Autodesk Fusion 360 part; units mm, degrees
sketch "Sketch1" plane through (0, 0, 0) normal (0, 1, 0) x (1, 0, 0)
  line L0 (0, -1) -> (0, 0)
  line L1 (12, 0) -> (12, 1)
  line L2 (12, 1) -> (13, 1)
  line L3 (2, -1.5) -> (2, -2.5)
  line L4 (2, -2.5) -> (1, -2.5)
  line L5 (2, -1.5) -> (3, -1.5)
  line L6 (4.5, -1.5) -> (4.5, -8.5)
  line L7 (3, -8.5) -> (3, -1.5)
  line L8 (4.5, -1.5) -> (10.5, -1.5)
  line L9 (12, -1.5) -> (12, -8.5)
  line L10 (10.5, -8.5) -> (10.5, -1.5)
  line L11 (17.5, -10) -> (3, -10)
  line L12 (3, -10) -> (3, -8.5)
  line L13 (4.5, -8.5) -> (10.5, -8.5)
  line L14 (12, -8.5) -> (17.5, -8.5)
  line L15 (1, -2.5) -> (1, -1)
  line L16 (1, -1) -> (0, -1)
  line L17 (12, -1.5) -> (13, -1.5)
  line L18 (13, -1.5) -> (13, 1)
  line L19 (12, 0) -> (0, 0)
  line L20 (23, -1.5) -> (23, -8.5)
  line L21 (22, -1.5) -> (22, 1)
  line L22 (32, -8.5) -> (32, -1.5)
  line L23 (30.5, -8.5) -> (24.5, -8.5)
  line L24 (30.5, -1.5) -> (24.5, -1.5)
  line L25 (32, -10) -> (32, -8.5)
  line L26 (23, 0) -> (23, 1)
  line L27 (33, -1.5) -> (32, -1.5)
  line L28 (23, 1) -> (22, 1)
  line L29 (34, -2.5) -> (34, -1)
  line L30 (24.5, -8.5) -> (24.5, -1.5)
  line L31 (23, 0) -> (35, 0)
  line L32 (23, -1.5) -> (22, -1.5)
  line L33 (34, -1) -> (35, -1)
  line L34 (30.5, -1.5) -> (30.5, -8.5)
  line L35 (33, -1.5) -> (33, -2.5)
  line L36 (35, -1) -> (35, 0)
  line L37 (23, -8.5) -> (17.5, -8.5)
  line L38 (17.5, -10) -> (32, -10)
  line L39 (33, -2.5) -> (34, -2.5)
  point P0 (35, 0)
  dimension "d2" = 1
  dimension "d9" = 1
  dimension "d10" = 1.5
  dimension "d11" = 7
  dimension "d12" = 6
  dimension "d13" = 1.5
  dimension "d14" = 7
  dimension "d15" = 14.5
  dimension "d16" = 1.5
extrude "Extrude1" add sketch "Sketch1" along normal blind 5
extrude "Extrude2" add 1 faces at (10.3333, 5, 9.5) along direction (0, 1, 0) blind 95
extrude "Extrude3" cut 1 faces at (1.6667, 66.6667, 2.5) along direction (0, 0, -1) blind 1
extrude "Extrude4" add 1 faces at (1, 66.6667, 1.3333) along direction (-1, 0, 0) blind 1
extrude "Extrude5" cut 1 faces at (33.3333, 33.3333, 2.5) along direction (0, 0, -1) blind 1
extrude "Extrude6" add 1 faces at (34, 66.6667, 1.3333) along direction (1, 0, 0) blind 1
extrude "Extrude7" add 1 faces at (13, 33.3333, 0.6667) along direction (1, 0, 0) blind 1
extrude "Extrude8" cut 1 faces at (12, 66.6667, -0.3333) along direction (1, 0, 0) blind 1
extrude "Extrude9" add 1 faces at (22, 33.3333, 0.6667) along direction (-1, 0, 0) blind 1
extrude "Extrude10" cut 1 faces at (23, 33.3333, -0.3333) along direction (-1, 0, 0) blind 1
extrude "Extrude11" add 1 faces at (13.3333, 66.6667, -1) along direction (0, 0, -1) blind 1
extrude "Extrude12" add 1 faces at (21.6667, 66.6667, -1) along direction (0, 0, -1) blind 1
extrude "Extrude13" add 1 faces at (14, 33.3333, -0.8333) along direction (1, 0, 0) blind 0.5
extrude "Extrude14" add 1 faces at (21, 66.6667, 0.3333) along direction (-1, 0, 0) blind 0.5
The listing builds one solid part. Answer for the finished solid, in the listing's coordinates (mm). A direction names the side the tool comes from. Give positions to 0.01 mm unless a question says otherwise; leave off trailing zeros. Order: outer loops, then holes, each group sorted by start corner. A loop starts at its lowest first (then second) coordinate and runs counter-clockwise, first axis right, second up.
Item 1: The part is cut by section C-C, the plane y = 13.5. Give the vertices of the cut face in (x, z).
From the geometry:
outline: (0, 0) - (13, 0) - (13, -2) - (14.5, -2) - (14.5, 1.5) - (12, 1.5) - (12, 8.5) - (23, 8.5) - (23, 1.5) - (20.5, 1.5) - (20.5, -2) - (22, -2) - (22, 0) - (35, 0) - (35, 1.5) - (32, 1.5) - (32, 10) - (3, 10) - (3, 1.5) - (0, 1.5) - close; hole (4.5, 1.5) - (10.5, 1.5) - (10.5, 8.5) - (4.5, 8.5) - close; hole (24.5, 1.5) - (30.5, 1.5) - (30.5, 8.5) - (24.5, 8.5) - close
Item 2: The part is cut by section D-D, the plane x = 18. Give the vertices of the cut face in (y, z).
From the geometry:
outline: (0, 8.5) - (100, 8.5) - (100, 10) - (0, 10) - close
Item 3: The part is cut by section A-A, the plane x = 6.5. Give the vertices of the cut face in (y, z).
From the geometry:
outline: (0, 0) - (100, 0) - (100, 1.5) - (0, 1.5) - close; (0, 8.5) - (100, 8.5) - (100, 10) - (0, 10) - close
Item 4: Given pin 1 Ø6.5 at (x, y) = (9, 72) entering from -Z; pin 2 Ø1 at (y, z) = (34.5, 6.5) entering from -X; pin 3 Ø0.6 at (y, z) = (63.5, -0.5) entering from +X, each flat-ended and moving along its own axis, determine where each tip first touches the part or whether it passes through.
From the geometry:
pin 1: stops at z = 0
pin 2: stops at x = 3
pin 3: stops at x = 22
Item 5: For a pull along Z with two mould halves and no side action, classify faces 5 (the face through (13, 51, 1.5)), 6 (the face through (17, 49, 10)), 7 (the face through (24, 0, 5)) as pulls with the +Z half, pulls with the -Z half, needs draft (parallel to the pull), parting line crosses it, or undercut.
From the geometry:
face 5: undercut
face 6: pulls with the +Z half
face 7: needs draft
Item 6: Which of the six approach directions +Z, -Z, +X, -X, +Y, -Y give full straight-line access (tool end or side, diameter ignored) to faces 1 (the face through (33, 51, 1.5)), 2 (the face through (20.5, 51, 0)), 3 (the face through (7, 49, 0)), 4 (the face through (22, 51, 1.5))?
From the geometry:
face 1: +Z, +X, +Y, -Y
face 2: -Z, +Y, -Y
face 3: -Z, -X, +Y, -Y
face 4: +Y, -Y
Item 7: Find the intervals of material crossed by probe 1 along X at (y, z) = (13.5, 6.5); probe 2 along X at (y, z) = (66, 0.25); probe 3 along Z at (x, y) = (10, 94.5), in increasing order.
From the geometry:
probe 1: x = 3 to 4.5, 10.5 to 12, 23 to 24.5, 30.5 to 32
probe 2: x = 0 to 14.5, 20.5 to 35
probe 3: z = 0 to 1.5, 8.5 to 10
Item 8: The part is cut by section B-B, the plane z = 6. Give the vertices of the cut face in (x, y), and give its area (3 significant figures).
From the geometry:
outline: (3, 0) - (4.5, 0) - (4.5, 100) - (3, 100) - close; (10.5, 0) - (12, 0) - (12, 100) - (10.5, 100) - close; (23, 0) - (24.5, 0) - (24.5, 100) - (23, 100) - close; (30.5, 0) - (32, 0) - (32, 100) - (30.5, 100) - close
area: 600 mm2
